```python
from build123d import *

# Parameters (mm, degrees)
BOSS_EXTRUDE1_DEPTH = 1317.1
CUT_EXTRUDE3_DEPTH  = 1388.288687357
BOSS_EXTRUDE5_DEPTH = 120
BOSS_EXTRUDE6_DEPTH = 30
BOSS_EXTRUDE7_START = -30
BOSS_EXTRUDE7_DEPTH = 30


with BuildPart() as part:
    # Sketch4 → Boss-Extrude1 (new body)
    with BuildSketch(Plane(origin=(0, 0, 0), x_dir=(0, 0, -1), z_dir=(1, 0, 0))):
        with BuildLine():
            Line((-159.891789037, -100.950379886), (-425.791789037, -100.950379886))
            Line((-425.791789037, -100.950379886), (-425.791789037, -77.297586412))
            Line((-425.791789037, -77.297586412), (-160.824878808, -77.297586412))
            ThreePointArc((-160.824878808, -77.297586412), (-71.405126121, -52.440077817), (-7.642881742, 15))
            Line((-7.642881742, 15), (0, 0))
            ThreePointArc((0, 0), (-65.345023624, -73.601000579), (-159.891789037, -100.950379886))
        make_face()
    extrude(amount=BOSS_EXTRUDE1_DEPTH)

    # Sketch10 → Cut-Extrude3 (cut, through all)
    with BuildSketch(Plane(origin=(0, -77.297586412, 0), x_dir=(1, 0, 0), z_dir=(0, 1, 0))):
        Polygon((0, -425.791789037), (478.6, -425.791789037), (0, -160.824878808), align=None)
        Polygon((1317.1, -160.824878808), (838.6, -425.791789037), (1317.1, -425.791789037), align=None)
    extrude(amount=-CUT_EXTRUDE3_DEPTH, mode=Mode.SUBTRACT)

    # Sketch11 → Boss-Extrude5 (add)
    with BuildSketch(Plane(origin=(0, -77.297586412, 0), x_dir=(1, 0, 0), z_dir=(0, 1, 0))):
        Polygon((838.6, -425.791789037), (808.6, -425.791789037), (1287.1, -160.824878808), (1317.1, -160.824878808), align=None)
        Polygon((478.6, -425.791789037), (508.6, -425.791789037), (30.1, -160.824878808), (0.1, -160.824878808), align=None)
    extrude(amount=BOSS_EXTRUDE5_DEPTH)

    # Sketch13 → Boss-Extrude6 (add)
    with BuildSketch(Plane(origin=(0, 0, 0), x_dir=(0, 0, -1), z_dir=(1, 0, 0))):
        with BuildLine():
            Line((-7.642881742, 15), (-160.824878808, 42.702413588))
            Line((-160.824878808, 42.702413588), (-160.824878808, -77.297586412))
            ThreePointArc((-160.824878808, -77.297586412), (-71.405126121, -52.440077817), (-7.642881742, 15))
        make_face()
    extrude(amount=BOSS_EXTRUDE6_DEPTH)

    # Sketch12 → Boss-Extrude7 (add)
    with BuildSketch(Plane(origin=(1317.1, 0, 0), x_dir=(0, 0, -1), z_dir=(1, 0, 0)).offset(BOSS_EXTRUDE7_START)):
        with BuildLine():
            Line((-7.642881742, 15), (-160.824878808, 42.702413588))
            Line((-160.824878808, 42.702413588), (-160.824878808, -77.297586412))
            ThreePointArc((-160.824878808, -77.297586412), (-71.405126121, -52.440077817), (-7.642881742, 15))
        make_face()
    extrude(amount=BOSS_EXTRUDE7_DEPTH)


solid = part.part
```
Work out the finished part from the listing and answer in its coordinate system (mm). A direction names the side the tool comes from. Give positions to 0.01 mm unless a question says otherwise; leave off trailing zeros. Loops run counter-clockwise (first coordinate to the right, second up) from the corner with the lowest first, then second, coordinate; pieces in that order, holes last. Notation, with made-up numbers: M 58.5,62.5 L 74.5,62.5 A17 cw 74.5,91.5 Z; hole C -28.75,0 d7. An arc over 180 degrees is marked long. One line per item, written item: value. Start each with the question number.
1. Find section A-A (x = 861.5). Give the vertices of the cut face in (y, z), and give its area (3 significant figures).
2. Find section B-B (y = -21). Give the vertices of the cut face in (x, z).
3. Find section D-D (x = 80). Give the vertices of the cut face in (y, z).
4. Which of the six approach directions +Z, -Z, +X, -X, +Y, -Y give full straight-line access (tool end or side, diameter ignored) to faces 4 (the face through (1287.1, -16, 102)), 5 (the face through (1301.89, 28.657, 83.162))?
5. Find section C-C (z = 64). Give the vertices of the cut face in (x, y).
6. Each of these flat-tipped pins is pushed along its axis until it touches: P1, Ø6, axis at x = 1012.5, y = -37, coming from the +Z side; P2, Ø4, axis at x = 330, y = -19, coming from the +Z side; P3, Ø3, axis at x = 681.5, z = 342, coming from the +Y side. Where does it stop, or does it pass through?
7. Determine the mould class of faces 1 (the face through (1081.2, -30.13, 291.454)), 2 (the face through (1064, 42.702, 293)), 3 (the face through (650, -77.298, 266)) for opening direction X: released by +X, released by -X, zero draft, split by the parting line, or undercut.
8. Find the intervals of material crossed by probe 1 along X at (y, z) = (-6.5, 156.5); probe 2 along Y at (x, z) = (859, 316.5); probe 3 along Z at (x, y) = (1044.5, -62), in increasing order.
Reported:
1. outline: M -100.95,159.89 A177.1 ccw 0,0 L 15,7.64 A173.26 cw -77.3,160.82 L -77.3,396.5 L 42.7,396.5 L 42.7,413.11 L -100.95,413.11 Z
1. area: 11,900 mm²
2. outline: M 0,11.82 L 1317.1,11.82 L 1317.1,160.82 L 838.6,425.79 L 808.6,425.79 L 1287.1,160.82 L 1287.1,33 L 30,33 L 30,160.82 L 30.1,160.82 L 508.6,425.79 L 478.6,425.79 L 0.1,160.82 L 0,160.82 Z
3. outline: M -100.95,159.89 A177.1 ccw 0,0 L 15,7.64 A173.26 cw -77.3,160.82 L -77.3,188.46 L 42.7,188.46 L 42.7,205.07 L -77.3,205.07 L -77.3,205.12 L -100.95,205.12 Z
4. face 4: +Y
4. face 5: -Z, +X, -X, +Y
5. outline: M 0,-72.74 L 1317.1,-72.74 L 1317.1,25.19 L 1287.1,25.19 L 1287.1,-47.72 L 30,-47.72 L 30,25.19 L 0,25.19 Z
6. P1: stops at z = 331.16
6. P2: stops at z = 344.61
6. P3: stops at y = -77.3
7. face 1: released by +X
7. face 2: zero draft
7. face 3: undercut
8. probe 1: x = 0 to 30, 1287.1 to 1317.1
8. probe 2: y = -100.95 to -77.3
8. probe 3: z = 49.08 to 89.64, 295.16 to 311.78
